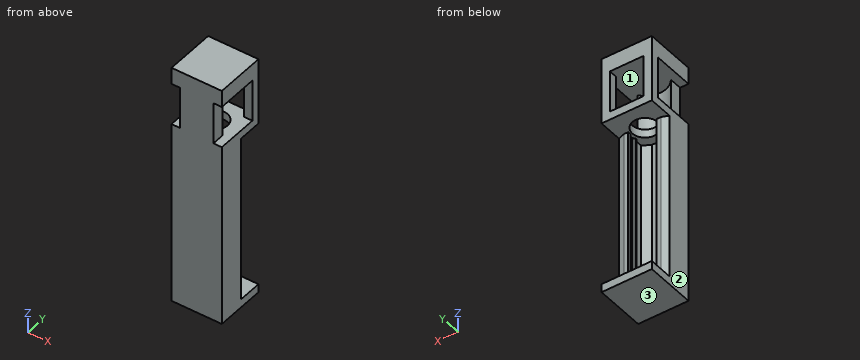
```python
from build123d import *

# Parameters (mm, degrees)
SKETCH1_W           = 60
SKETCH1_H           = 60
BOSS_EXTRUDE1_DEPTH = 80
CUT_EXTRUDE3_DEPTH  = 60
SKETCH6_W           = 60
SKETCH6_H           = 60
BOSS_EXTRUDE3_DEPTH = 10
SKETCH7_R           = 15
CUT_EXTRUDE4_DEPTH  = 10
BOSS_EXTRUDE4_DEPTH = 200
SKETCH10_W          = 60
SKETCH10_H          = 10
BOSS_EXTRUDE5_DEPTH = 60


with BuildPart() as part:
    # Sketch1 → Boss-Extrude1 (new body)
    with BuildSketch(Plane.XY):
        Rectangle(SKETCH1_W, SKETCH1_H)
    extrude(amount=BOSS_EXTRUDE1_DEPTH)

    # Sketch5 → Cut-Extrude3 (cut)
    with BuildSketch(Plane(origin=(0, 0, 0), x_dir=(-1, 0, 0), z_dir=(0, 0, -1))):
        with BuildLine():
            Line((20, 30), (-20, 30))
            Line((-20, 30), (-20, 20))
            Line((-20, 20), (-30, 20))
            Line((-30, 20), (-30, -30))
            Line((-30, -30), (-20, -30))
            Line((-20, -30), (-20, -15))
            ThreePointArc((-20, -15), (0, -25), (20, -15))
            Line((20, -15), (20, -30))
            Line((20, -30), (30, -30))
            Line((30, -30), (30, 20))
            Line((30, 20), (20, 20))
            Line((20, 20), (20, 30))
        make_face()
    extrude(amount=-CUT_EXTRUDE3_DEPTH, mode=Mode.SUBTRACT)

    # Sketch6 → Boss-Extrude3 (add)
    with BuildSketch(Plane(origin=(0, 0, 0), x_dir=(-1, 0, 0), z_dir=(0, 0, -1))):
        Rectangle(SKETCH6_W, SKETCH6_H)
    extrude(amount=-BOSS_EXTRUDE3_DEPTH)

    # Sketch7 → Cut-Extrude4 (cut)
    with BuildSketch(Plane(origin=(0, 0, 0), x_dir=(-1, 0, 0), z_dir=(0, 0, -1))):
        Circle(SKETCH7_R)
    extrude(amount=-CUT_EXTRUDE4_DEPTH, mode=Mode.SUBTRACT)

    # Sketch8 → Boss-Extrude4 (add)
    with BuildSketch(Plane(origin=(0, 0, 0), x_dir=(-1, 0, 0), z_dir=(0, 0, -1))):
        Polygon((-30, -25), (-10, -25), (-19, -19.803847577), (-19, -11.803847577), (-17, -9.803847577), (-17, -7.803847577), (-19, -5.803847577), (-19, 0.196152423), (-17, 0.196152423), (-17, 4.196152423), (-22, 4.196152423), (-30, 1.196152423), align=None)
        Polygon((19, -19.803847577), (10, -25), (30, -25), (30, 1.196152423), (22, 4.196152423), (17, 4.196152423), (17, 0.196152423), (19, 0.196152423), (19, -5.803847577), (17, -7.803847577), (17, -9.803847577), (19, -11.803847577), align=None)
        Polygon((10, -25), (0, -25), (0, -30), (30, -30), (30, -25), align=None)
        Polygon((0, -30), (0, -25), (-10, -25), (-30, -25), (-30, -30), align=None)
    extrude(amount=BOSS_EXTRUDE4_DEPTH)

    # Sketch10 → Boss-Extrude5 (add)
    with BuildSketch(Plane.XZ.offset(30)):
        with Locations((0, -205)):
            Rectangle(SKETCH10_W, SKETCH10_H)
    extrude(amount=-BOSS_EXTRUDE5_DEPTH)


solid = part.part
```
Can you work these out from the model? Positions are in its coordinate system, mm. Face numbers are marked on the shaded views. Coordinates: 2 decimals unless noted, no trailing zeros. Loops run counter-clockwise (first coordinate to the right, second up) from the corner with the lowest first, then second, coordinate; pieces in that order, holes last.
1) I need wall thicknesses on probe 1 along Z at (x, y) = (-26, 7); probe 2 along Z at (x, y) = (23.5, -16); probe 3 along Z at (x, y) = (-26.5, 24.5). Which ranges of each line are inside material? Lowest first, please.
2) Imagine slicing it at D-D on z = -84.5. List the corners of the cut face in (x, y) for me, plus the area to 3 significant figures.
3) Imagine slicing it at A-A on x = 0. List the corners of the cut face in (y, z) for me, plus the area to 3 significant figures.
4) Imagine slicing it at B-B on z = 41. List the corners of the cut face in (x, y) for me, plus the area to 3 significant figures.
5) Imagine slicing it at C-C on y = 9. List the corners of the cut face in (x, z) for me, plus the area to 3 significant figures.
6) Thinking about a two-plate mould opening in Z: for the marked faces 1, 2 and 3, which applies, pulls with the +Z half, pulls with the -Z half, needs draft (parallel to the pull), parting line crosses it, or undercut?
7) For pin 1 (7.5 mm diameter, centred on y = -23.5, z = 40, fed in from +X); pin 2 (4 mm diameter, centred on x = 19, z = -65, fed in from +Y); pin 3 (12 mm diameter, centred on y = 2, z = -84, fed in from +X); pin 4 (7.5 mm diameter, centred on y = -21, z = 35, fed in from -X), each with a flat end and sliding along its axis, tell me the tip position at first contact or that it passes through.
Completed:
1. probe 1: z = -210 to -200, 0 to 10, 60 to 80
1. probe 2: z = -210 to 10, 60 to 80
1. probe 3: z = -210 to -200, 0 to 80
2. outline: (-30, -30) - (30, -30) - (30, 1.2) - (22, 4.2) - (17, 4.2) - (17, 0.2) - (19, 0.2) - (19, -5.8) - (17, -7.8) - (17, -9.8) - (19, -11.8) - (19, -19.8) - (10, -25) - (-10, -25) - (-19, -19.8) - (-19, -11.8) - (-17, -9.8) - (-17, -7.8) - (-19, -5.8) - (-19, 0.2) - (-17, 0.2) - (-17, 4.2) - (-22, 4.2) - (-30, 1.2) - close
2. area: 997 mm2
3. outline: (-30, -210) - (30, -210) - (30, -200) - (-25, -200) - (-25, 0) - (-15, 0) - (-15, 10) - (-25, 10) - (-25, 60) - (30, 60) - (30, 80) - (-30, 80) - close; (15, 0) - (30, 0) - (30, 10) - (15, 10) - close
3. area: 3,350 mm2
4. outline: (-30, 20) - (-20, 20) - (-20, 30) - (-30, 30) - close; (-20, -30) - (20, -30) - (20, -15) arc R25 cw to (-20, -15) - close; (20, 20) - (30, 20) - (30, 30) - (20, 30) - close
4. area: 520 mm2
5. outline: (-30, -210) - (30, -210) - (30, -200) - (-30, -200) - close; (-30, 0) - (-12, 0) - (-12, 10) - (-30, 10) - close; (-30, 60) - (30, 60) - (30, 80) - (-30, 80) - close; (12, 0) - (30, 0) - (30, 10) - (12, 10) - close
5. area: 2,160 mm2
6. face 1: undercut
6. face 2: needs draft
6. face 3: pulls with the -Z half
7. pin 1: stops at x = 20
7. pin 2: stops at y = 4.2
7. pin 3: stops at x = 30
7. pin 4: stops at x = -20
